For this review, take the finished solid that the model builds, in its own axes (mm). Coordinates: 2 decimals unless noted, no trailing zeros. Write each loop counter-clockwise with the first axis right and the second up, starting at its lowest first coordinate (ties: lowest second). Pieces come first, ordered by that corner, then holes.
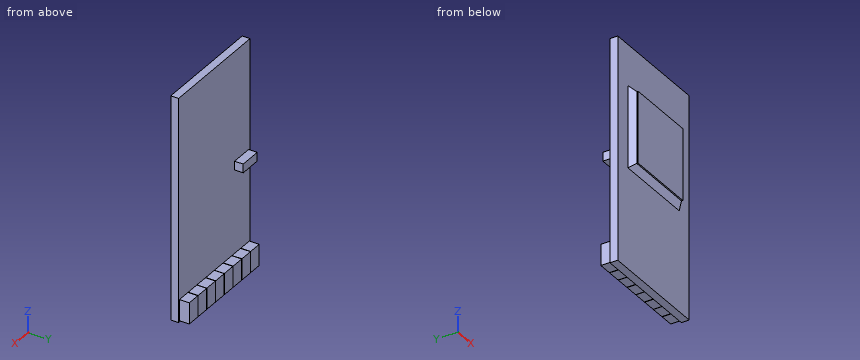
```python
from build123d import *

# Parameters (mm, degrees)
SKETCH1_W           = 23
SKETCH1_H           = 45
BOSS_EXTRUDE1_DEPTH = 1.5875
SKETCH2_W           = 16.5
SKETCH2_H           = 16.5
BOSS_EXTRUDE2_DEPTH = 1.14
BOSS_EXTRUDE2_TAPER = 42.37
SKETCH3_W           = 14.42
SKETCH3_H           = 14.42
BOSS_EXTRUDE3_DEPTH = 0.26
SKETCH4_W           = 2.75
SKETCH4_H           = 4.25
BOSS_EXTRUDE4_DEPTH = 2
SKETCH5_W           = 4.5
SKETCH5_H           = 1.75
BOSS_EXTRUDE5_DEPTH = 1.75


with BuildPart() as part:
    # Sketch1 → Boss-Extrude1 (new body)
    with BuildSketch(Plane(origin=(0, 0, 0), x_dir=(1, 0, 0), z_dir=(0, 1, 0))):
        with Locations((11.5, 22.5)):
            Rectangle(SKETCH1_W, SKETCH1_H)
    extrude(amount=BOSS_EXTRUDE1_DEPTH)

    # Sketch2 → Boss-Extrude2 (add)
    with BuildSketch(Plane.XZ):
        with Locations((11.5, -16.5)):
            Rectangle(SKETCH2_W, SKETCH2_H)
    extrude(amount=BOSS_EXTRUDE2_DEPTH, taper=BOSS_EXTRUDE2_TAPER)

    # Sketch3 → Boss-Extrude3 (add)
    with BuildSketch(Plane.XZ.offset(1.14)):
        with Locations((11.5, -16.5)):
            Rectangle(SKETCH3_W, SKETCH3_H)
    extrude(amount=BOSS_EXTRUDE3_DEPTH)

    # Sketch4 → Boss-Extrude4 (add)
    with BuildSketch(Plane(origin=(0, 1.5875, 0), x_dir=(1, 0, 0), z_dir=(0, 1, 0))):
        with Locations((4.446, 42.625)):
            Rectangle(SKETCH4_W, SKETCH4_H)
        with Locations((1.625, 42.625)):
            Rectangle(SKETCH4_W, SKETCH4_H)
        with Locations((7.267, 42.625)):
            Rectangle(SKETCH4_W, SKETCH4_H)
        with Locations((10.088, 42.625)):
            Rectangle(SKETCH4_W, SKETCH4_H)
        with Locations((12.909, 42.625)):
            Rectangle(SKETCH4_W, SKETCH4_H)
        with Locations((15.73, 42.625)):
            Rectangle(SKETCH4_W, SKETCH4_H)
        with Locations((18.551, 42.625)):
            Rectangle(SKETCH4_W, SKETCH4_H)
        with Locations((21.372, 42.625)):
            Rectangle(SKETCH4_W, SKETCH4_H)
    extrude(amount=BOSS_EXTRUDE4_DEPTH)

    # Sketch5 → Boss-Extrude5 (add)
    with BuildSketch(Plane(origin=(0, 1.5875, 0), x_dir=(1, 0, 0), z_dir=(0, 1, 0))):
        with Locations((2.75, 22.875)):
            Rectangle(SKETCH5_W, SKETCH5_H)
    extrude(amount=BOSS_EXTRUDE5_DEPTH)


solid = part.part
```
Q1. Add section A-A (y = 2.8). Give the number of separate pieces and of enclosed holes in the cut face, then the cut area to 3 significant figures.
Ans:
separate pieces: 9
enclosed holes: 0
area: 101 mm2
Q2. Add section B-B (z = -7). State the section outline as (x, y) points.
Ans:
outline: (0, 0) - (23, 0) - (23, 1.59) - (0, 1.59) - close
Q3. Clearance check with flat-ended pins moving along their axes: pin 1 Ø11.5 at (x, z) = (10.5, -24) entering from +Y; pin 2 Ø1.6 at (y, z) = (3, -42.5) entering from -X; pin 3 Ø1.9 at (y, z) = (2.5, -22.5) entering from -X; pin 4 Ø1.6 at (y, z) = (3, -42.5) entering from +X. State where each tip first meets the part, or that it passes through.
Ans:
pin 1: stops at y = 3.34
pin 2: stops at x = 0.25
pin 3: stops at x = 0
pin 4: stops at x = 22.75
Q4. For probe 1 along Z at (x, y) = (2.75, 2.5); probe 2 along Z at (x, y) = (22, 2.4); probe 3 along Y at (x, z) = (7, -7.5), list the stretches that pass through material, from the lowest coordinate up.
Ans:
probe 1: z = -44.75 to -40.5, -23.75 to -22
probe 2: z = -44.75 to -40.5
probe 3: y = 0 to 1.59
